Part model, mm, in its own coordinate system. A direction names the side the tool comes from. Round coordinates to 2 decimals unless told otherwise and drop trailing zeros. Write each loop counter-clockwise with the first axis right and the second up, starting at its lowest first coordinate (ties: lowest second). Pieces come first, ordered by that corner, then holes. Notation, with made-up numbers: M -35.5,12 L -5.5,12 A23 cw -5.5,36 Z; hole C 21.25,76 d3. An arc over 180 degrees is marked long. Use a Markdown table: item, result. Add a question column.
1) Slice it at D-D on x = -5.5. Write the cut outline in (y, z), plus the area to 3 significant figures.
2) Slice it at B-B on z = -4.75. Write the cut outline in (x, y).
3) Two-plate mould, pull along X, no slides. Class faces 1 (the face through (4.7, 70, -0.3)), 2 (the face through (11.377, 61.774, -0.246)), 3 (the face through (21.819, 35, -6)): released by +X, released by -X, zero draft, split by the parting line, or undercut.
4) Slice it at C-C on y = 13. Write the cut outline in (x, z), plus the area to 3 significant figures.
5) Wall check: probe 1 along Y at (x, z) = (-11.95, -7); probe 2 along X at (y, z) = (44, -2.25); probe 3 along Z at (x, y) = (17, 47). Give the ranges that are in metal, low to high.
6) Which spindle directions (+Z, -Z, +X, -X, +Y, -Y) get a long thin tool onto all of the face, cutting with end or side? Do faces 4 (the face through (21.566, 46.464, -6.675)), 5 (the face through (-11.681, 35, -6)). Say none if no direction does.
7) Drop flat-ended pins along their axis: P1, Ø2.5, axis at y = 25, z = -7, coming from the +X side; P2, Ø3, axis at x = 1, y = 61.5, coming from the -Z side. Give the stop position or say it passes through.
8) Slice it at A-A on y = 45. Write the cut outline in (x, z), plus the area to 3 significant figures.
```python
from build123d import *

# Parameters (mm, degrees)
BRIDA_BASE1_DEPTH     = 70
CROQUIS5_R            = 2.5
CROQUIS5_R_2          = 1.125
CROQUIS5_R_3          = 1.5
CORTAR_EXTRUIR1_DEPTH = 10
CROQUIS6_R            = 1.5
CORTAR_EXTRUIR3_DEPTH = 79.74007874


# Sheet-metal steps are written as plain solids
with BuildPart() as part:
    # Croquis1 → Brida base1 (new body)
    with BuildSketch(Plane(origin=(0, 0, 0), x_dir=(1, 0, 0), z_dir=(0, 1, 0))):
        with BuildLine():
            Line((-12.180744501, 12), (-12.180744501, 1))
            ThreePointArc((-12.180744501, 1), (-11.887851282, 0.292893219), (-11.180744501, 0))
            Line((-11.180744501, 0), (20.819255499, 0))
            ThreePointArc((20.819255499, 0), (21.52636228, 0.292893219), (21.819255499, 1))
            Line((21.819255499, 1), (21.819255499, 12))
            Line((21.819255499, 12), (21.319255499, 12))
            Line((21.319255499, 12), (21.319255499, 1))
            ThreePointArc((21.319255499, 1), (21.17280889, 0.646446609), (20.819255499, 0.5))
            Line((20.819255499, 0.5), (-11.180744501, 0.5))
            ThreePointArc((-11.180744501, 0.5), (-11.534297891, 0.646446609), (-11.680744501, 1))
            Line((-11.680744501, 1), (-11.680744501, 12))
            Line((-11.680744501, 12), (-12.180744501, 12))
        make_face()
    extrude(amount=BRIDA_BASE1_DEPTH)

    # Croquis5 → Cortar-Extruir1 (cut)
    with BuildSketch(Plane.XY):
        with Locations((4.819255499, 35)):
            Circle(CROQUIS5_R)
        with Locations((-1.430744501, 35)):
            Circle(CROQUIS5_R_2)
        with Locations(Location((11.069255499, 35, 0), (0, 0, 180))):
            Circle(CROQUIS5_R_2)
        with Locations((-2.430744501, 60.4433725)):
            Circle(CROQUIS5_R_3)
        with Locations(Location((12.069255499, 60.4433725, 0), (0, 0, 180))):
            Circle(CROQUIS5_R_3)
    extrude(amount=-CORTAR_EXTRUIR1_DEPTH, mode=Mode.SUBTRACT)

    # Croquis6 → Cortar-Extruir3 (cut, through all)
    with BuildSketch(Plane.ZY.offset(12.180744501)):
        with Locations(Location((-7, 45, 0), (0, 0, 180))):
            Circle(CROQUIS6_R)
        with Locations((-7, 25)):
            Circle(CROQUIS6_R)
        with Locations((-7, 5)):
            Circle(CROQUIS6_R)
        with Locations(Location((-7, 65, 0), (0, 0, 180))):
            Circle(CROQUIS6_R)
    extrude(amount=-CORTAR_EXTRUIR3_DEPTH, mode=Mode.SUBTRACT)


solid = part.part
```
Entries:
| question | item | result |
|---|---|---|
| 1 | outline | M 0,-0.5 L 70,-0.5 L 70,0 L 0,0 Z |
| 1 | area | 35.0 mm^2 |
| 2 | outline | M -12.18,0 L -11.68,0 L -11.68,70 L -12.18,70 Z; M 21.32,0 L 21.82,0 L 21.82,70 L 21.32,70 Z |
| 3 | face 1 | zero draft |
| 3 | face 2 | undercut |
| 3 | face 3 | released by +X |
| 4 | outline | M -12.18,-12 L -11.68,-12 L -11.68,-1 A0.5 cw -11.18,-0.5 L 20.82,-0.5 A0.5 cw 21.32,-1 L 21.32,-12 L 21.82,-12 L 21.82,-1 A1 ccw 20.82,0 L -11.18,0 A1 ccw -12.18,-1 Z |
| 4 | area | 28.2 mm^2 |
| 5 | probe 1 | y = 0 to 3.5, 6.5 to 23.5, 26.5 to 43.5, 46.5 to 63.5, 66.5 to 70 |
| 5 | probe 2 | x = -12.18 to -11.68, 21.32 to 21.82 |
| 5 | probe 3 | z = -0.5 to 0 |
| 6 | face 4 | +X, -X |
| 6 | face 5 | -Z, +Y, -Y |
| 7 | P1 | passes through |
| 7 | P2 | stops at z = -0.5 |
| 8 | outline | M -12.18,-12 L -11.68,-12 L -11.68,-8.5 L -12.18,-8.5 Z; M -12.18,-5.5 L -11.68,-5.5 L -11.68,-1 A0.5 cw -11.18,-0.5 L 20.82,-0.5 A0.5 cw 21.32,-1 L 21.32,-5.5 L 21.82,-5.5 L 21.82,-1 A1 ccw 20.82,0 L -11.18,0 A1 ccw -12.18,-1 Z; M 21.32,-12 L 21.82,-12 L 21.82,-8.5 L 21.32,-8.5 Z |
| 8 | area | 25.2 mm^2 |
